```python
from build123d import *

# Parameters (mm, degrees)
BOSS_EXTRUDE1_DEPTH = 60
SKETCH6_W           = 104.365742104
SKETCH6_H           = 42.078428343
CUT_EXTRUDE1_DEPTH  = 60
SKETCH7_R           = 5
CUT_EXTRUDE2_DEPTH  = 80
SKETCH8_R           = 5
CUT_EXTRUDE3_DEPTH  = 80


with BuildPart() as part:
    # Sketch1 → Boss-Extrude1 (new body)
    with BuildSketch(Plane.XY):
        with BuildLine():
            Line((-221.321453318, 37.052081842), (-74.563130632, 39.85043969))
            Line((-74.563130632, 39.85043969), (-53.022046647, 49.170731686))
            Line((-53.022046647, 49.170731686), (83.431852104, 44.510585688))
            Line((83.431852104, 44.510585688), (169.619936548, 0.125236974))
            ThreePointArc((169.619936548, 0.125236974), (179.310534794, -30.143946614), (149.041351206, -39.83454486))
            Line((149.041351206, -39.83454486), (113.217328202, -21.385802628))
            Line((113.217328202, -21.385802628), (-53.022046647, -36.262839488))
            Line((-53.022046647, -36.262839488), (-219.455881419, -39.436365998))
            ThreePointArc((-219.455881419, -39.436365998), (-232.557507777, -1.488943064), (-221.321453318, 37.052081842))
        make_face()
    extrude(amount=BOSS_EXTRUDE1_DEPTH)

    # Sketch6 → Cut-Extrude1 (cut)
    with BuildSketch(Plane(origin=(35.60593299, 69.14009348, 0), x_dir=(0.889035749, -0.457837785, 0), z_dir=(0.457837785, 0.889035749, 0))):
        with Locations((129.620714118, -29.693602711)):
            Rectangle(SKETCH6_W, SKETCH6_H)
    extrude(amount=-CUT_EXTRUDE1_DEPTH, mode=Mode.SUBTRACT)

    # Sketch7 → Cut-Extrude2 (cut)
    with BuildSketch(Plane.XY.offset(60)):
        with Locations((-201.23397976, 2.428743615)):
            Circle(SKETCH7_R)
    extrude(amount=-CUT_EXTRUDE2_DEPTH, mode=Mode.SUBTRACT)

    # Sketch8 → Cut-Extrude3 (cut)
    with BuildSketch(Plane.XY.offset(60)):
        with Locations((154.912488727, -17.513734237)):
            Circle(SKETCH8_R)
    extrude(amount=-CUT_EXTRUDE3_DEPTH, mode=Mode.SUBTRACT)


solid = part.part
```
The listing builds one solid part. Answer for the finished solid, in the listing's coordinates (mm). A direction names the side the tool comes from. Coordinates: 2 decimals unless noted, no trailing zeros. Loops run counter-clockwise (first coordinate to the right, second up) from the corner with the lowest first, then second, coordinate; pieces in that order, holes last. Notation, with made-up numbers: (78, 6.25) - (120, 6.25) arc R7 cw to (120, 19.25) - close; hole circle Ø7 at (-34.75, 11.25). An arc over 180 degrees is marked (long way). Use a Markdown table: item, result. Add a question column.
1) Given pin 1 (4 mm diameter, centred on y = 19, z = 20, fed in from -X); pin 2 (12 mm diameter, centred on x = 92, z = 31, fed in from -Y); pin 3 (4 mm diameter, centred on y = 21.5, z = 16, fed in from -X), each flat-ended and moving along its own axis, determine where each tip first touches the part or whether it passes through.
2) The part is cut by section D-D, the plane y = 13. Give the vertices of the cut face in (x, z), and give its area (3 significant figures).
3) The part is cut by section B-B, the plane z = 12.5. Give the vertices of the cut face in (x, y).
4) The mould has two halves that part along Z. Classify faces 4 (the flat face through (-63.943, 44.445, 29.58)), 5 (the flat face through (-22, 4, 0)), 6 (the flat face through (136, -8, 8.654)): released by +Z, released by -Z, zero draft, split by the parting line, or undercut.
5) Find the intervals of material crossed by line 1 (Z direction, x = 145, y = -5); line 2 (X direction, y = -13, z = 53); line 3 (X direction, y = 6.5, z = 18), in increasing order.
6) The part is cut by section C-C, the plane z = 55.5. Give the vertices of the cut face in (x, y).
7) The part is cut by section A-A, the plane y = -27.5. Give the vertices of the cut face in (x, z).
8) For faces 1 (the flat face through (81.036, -21.745, 29.399)), 2 (the flat face through (131.38, -30.74, 4.27)), 3 (the flat face through (97.193, 37.424, 29.58)), determine the directions among +Z, -Z, +X, -X, +Y, -Y from which every point of the face is accessible in a straight line to the end or side of a thin tool.
Here are the results:
| question | item | result |
|---|---|---|
| 1 | pin 1 | stops at x = -230.39 |
| 1 | pin 2 | stops at y = -2.14 |
| 1 | pin 3 | stops at x = -229.68 |
| 2 | outline | (-231.31, 0) - (144.62, 0) - (144.62, 8.65) - (93.8, 8.65) - (93.8, 50.73) - (144.62, 50.73) - (144.62, 60) - (-231.31, 60) - close |
| 2 | area | 20,400 mm^2 |
| 3 | outline | (-221.32, 37.05) arc R66.2 ccw to (-219.46, -39.44) - (-53.02, -36.26) - (85.21, -23.89) - (76.98, -19.66) - (104.45, 33.69) - (83.43, 44.51) - (-53.02, 49.17) - (-74.56, 39.85) - close; hole circle Ø10 at (-201.23, 2.43) |
| 4 | face 4 | zero draft |
| 4 | face 5 | released by -Z |
| 4 | face 6 | undercut |
| 5 | line 1 | z = 0 to 8.65, 50.73 to 60 |
| 5 | line 2 | x = -231.26 to 152.76, 157.06 to 180.73 |
| 5 | line 3 | x = -232.27 to -204.14, -198.33 to 90.45 |
| 6 | outline | (-221.32, 37.05) arc R66.2 ccw to (-219.46, -39.44) - (-53.02, -36.26) - (113.22, -21.39) - (149.04, -39.83) arc R22.47 ccw to (169.62, 0.13) - (83.43, 44.51) - (-53.02, 49.17) - (-74.56, 39.85) - close; hole circle Ø10 at (-201.23, 2.43); hole circle Ø10 at (154.91, -17.51) |
| 7 | outline | (-226.54, 0) - (44.9, 0) - (44.9, 60) - (-226.54, 60) - close; (125.09, 0) - (180.46, 0) - (180.46, 8.65) - (125.09, 8.65) - close; (125.09, 50.73) - (180.46, 50.73) - (180.46, 60) - (125.09, 60) - close |
| 8 | face 1 | +X |
| 8 | face 2 | +Z, -Z, -Y |
| 8 | face 3 | +Z, -Z, +X, +Y |
